```python
from build123d import *

# Parameters (mm, degrees)
F0_R        = 1.5
F1_DEPTH    = 10
F2_DEPTH    = 20
F4_R        = 1.6
F5_DEPTH    = 15
F6_T1_DEPTH = 40
F6_T3_DEPTH = 41.1
F6_T5_DEPTH = 35.7954738485


# Not quite as in the source:
# - a fillet or chamfer that OpenCascade refuses, or shapes differently, is made with other operations: its cross-section is extruded or revolved along the edge and cut away or added


with BuildPart() as f1:
    # F0 (on Top) → F1 (new body)
    with BuildSketch(Plane.XY):
        with BuildLine():
            Line((-15.25, 4.3355262056), (-20.5, 4.5))
            Line((-20.5, 4.5), (-20.5, -4.5))
            Line((-20.5, -4.5), (-10.9144737944, -4.5))
            Line((-10.9144737944, -4.5), (-10.9144737944, 0))
            ThreePointArc((-10.9144737944, 0), (-12.18432002, 3.06567998), (-15.25, 4.3355262056))
        make_face()
        with Locations((-15.25, 0)):
            Circle(F0_R, mode=Mode.SUBTRACT)
        Polygon((20.5, -8.5), (20.5, -4.5), (10.9144737944, -4.5), (-10.9144737944, -4.5), (-20.5, -4.5), (-20.5, -8.5), align=None)
        with BuildLine():
            Line((20.5, -4.5), (20.5, 4.5))
            Line((20.5, 4.5), (15.25, 4.3355262056))
            ThreePointArc((15.25, 4.3355262056), (12.18432002, 3.06567998), (10.9144737944, 0))
            Line((10.9144737944, 0), (10.9144737944, -4.5))
            Line((10.9144737944, -4.5), (20.5, -4.5))
        make_face()
        with Locations((15.25, 0)):
            Circle(F0_R, mode=Mode.SUBTRACT)
    extrude(amount=F1_DEPTH)


with BuildPart() as f2:
    # F0 (on Top) → F2 (new body)
    with BuildSketch(Plane.XY):
        Polygon((20.5, 7.6), (20.5, 4.5), (20.5, -4.5), (20.5, -8.5), (24, -8.5), (24, 0), (24, 7.6), align=None)
    extrude(amount=F2_DEPTH)


with BuildPart() as f1_1:
    add(f1.part)

    # F3: union F2
    add(f2.part)

    # F4 (on face) → F5 (join)
    with BuildSketch(Plane.XZ.offset(8.5)):
        with BuildLine():
            Line((24, 14), (24, 0))
            Line((24, 0), (50, 0))
            Line((50, 0), (50, 14))
            Line((50, 14), (50, 20))
            Line((50, 20), (43.5623936355, 20))
            Line((43.5623936355, 20), (43.5623936355, 14))
            Line((43.5623936355, 14), (43.5, 14))
            ThreePointArc((43.5, 14), (37, 7.5), (30.5, 14))
            Line((30.5, 14), (30.5, 20))
            Line((30.5, 20), (24, 20))
            Line((24, 20), (24, 14))
        make_face()
        with Locations((28, 14)):
            Circle(F4_R, mode=Mode.SUBTRACT)
        with Locations((46, 14)):
            Circle(F4_R, mode=Mode.SUBTRACT)
    extrude(amount=-F5_DEPTH)

    # F6: fillet of radius 5 on 5 edges, made by hand

    # F6_s2 → F6_t1 (cut)
    with BuildSketch(Plane.XZ.offset(-19)):
        with BuildLine():
            ThreePointArc((43.5623936355, 15), (45.0268597296, 18.5355339059), (48.5623936355, 20))
            Line((48.5623936355, 20), (43.5623936355, 20))
            Line((43.5623936355, 20), (43.5623936355, 15))
        make_face()
        with BuildLine():
            ThreePointArc((45, 20), (48.5355339059, 18.5355339059), (50, 15))
            Line((50, 15), (50, 20))
            Line((50, 20), (45, 20))
        make_face()
        with BuildLine():
            ThreePointArc((30.5, 15), (29.0355339059, 18.5355339059), (25.5, 20))
            Line((25.5, 20), (30.5, 20))
            Line((30.5, 20), (30.5, 15))
        make_face()
    extrude(amount=F6_T1_DEPTH, mode=Mode.SUBTRACT)

    # F6_s4 → F6_t3 (cut)
    with BuildSketch(Plane.XZ.offset(-20.1)):
        with BuildLine():
            ThreePointArc((20.5, 15), (21.9644660941, 18.5355339059), (25.5, 20))
            Line((25.5, 20), (20.5, 20))
            Line((20.5, 20), (20.5, 15))
        make_face()
    extrude(amount=F6_T3_DEPTH, mode=Mode.SUBTRACT)

    # F6_s6 → F6_t5 (cut)
    with BuildSketch(Plane.XY.offset(-12.8977369243)):
        with BuildLine():
            ThreePointArc((-20.5, -0.6590947697), (-18.9797396108, 2.9313665155), (-15.3434351037, 4.3384533725))
            Line((-15.3434351037, 4.3384533725), (-20.5, 4.5))
            Line((-20.5, 4.5), (-20.5, -0.6590947697))
        make_face()
    extrude(amount=F6_T5_DEPTH, mode=Mode.SUBTRACT)


solid = f1_1.part
```
Input: part model. Units: mm. Frame: model coordinates. A direction names the side the tool comes from. Round coordinates to 2 decimals unless told otherwise and drop trailing zeros. Loops run counter-clockwise (first coordinate to the right, second up) from the corner with the lowest first, then second, coordinate; pieces in that order, holes last. Notation, with made-up numbers: (-30.5, 1) -> (-20.5, 1) arc R21 ccw to (-20.5, 36) -> close; hole circle Ø6 at (89, 60.5). An arc over 180 degrees is marked (long way). Write each question's results on one line, items separated by ' | '.
1. Section C-C (x = 37). Return loops of the section in (y, z).
Geometry results:
outline: (-8.5, 0) -> (6.5, 0) -> (6.5, 7.5) -> (-8.5, 7.5) -> close
2. Set-up query: faces 1 (the face through (0, -5, 10)), 2 (the face through (-12.15, 3.03, 4.93)), 3 (the face through (44.42, -0.89, 17.8)). Return all of +Z, -Z, +X, -X, +Y, -Y with unobstructed straight access to the full face (end or side cutting, diameter ignored); none if empty.
Geometry results:
face 1: +Z, -X, +Y, -Y | face 2: +Z, -Z, +Y | face 3: +Z, +Y, -Y
3. Section A-A (z = 3.25). Return loops of the section in (x, y), and give its area (3 significant figures).
Geometry results:
outline: (-20.5, -8.5) -> (50, -8.5) -> (50, 6.5) -> (24, 6.5) -> (24, 7.6) -> (20.5, 7.6) -> (20.5, 4.5) -> (15.25, 4.34) arc R4.34 ccw to (10.91, 0) -> (10.91, -4.5) -> (-10.91, -4.5) -> (-10.91, 0) arc R4.34 ccw to (-15.25, 4.34) -> (-15.34, 4.34) arc R5 ccw to (-20.5, -0.66) -> close; hole circle Ø3 at (-15.25, 0); hole circle Ø3 at (15.25, 0) | area: 753 mm2
4. Section D-D (x = -7). Return loops of the section in (y, z), and give its area (3 significant figures).
Geometry results:
outline: (-8.5, 0) -> (-4.5, 0) -> (-4.5, 10) -> (-8.5, 10) -> close | area: 40.0 mm2
5. Section B-B (x = 28). Return loops of the section in (y, z), and give its area (3 significant figures).
Geometry results:
outline: (-8.5, 0) -> (6.5, 0) -> (6.5, 12.4) -> (-8.5, 12.4) -> close; (-8.5, 15.6) -> (6.5, 15.6) -> (6.5, 19.33) -> (-8.5, 19.33) -> close | area: 242 mm2
6. Ray query, line 1 (X direction, y = -4.25, z = 13); line 2 (Y direction, x = -15.25, z = 2); line 3 (X direction, y = 2, z = 14.75). Return the intervals inside material, ascending. Write a range as from..to.
Geometry results:
line 1: 20.5..26.75, 29.25..30.58, 43.42..44.75, 47.25..50 | line 2: -8.5..-1.5, 1.5..4.34 | line 3: 20.5..26.59, 29.41..30.5, 43.56..44.59, 47.41..50
7. First-contact query: P1, Ø1.5, axis at y = 5.5, z = 4.5, coming from the -X side; P2, Ø0.6, axis at y = 7, z = 9.5, coming from the +X side; P3, Ø1.8, axis at x = -15.25, y = 0, coming from the -Z side; P4, Ø5, axis at x = -1, z = 4.5, coming from the +Y side. Flat tips, straight axial feed; report the tip coordinate or a pass-through.
Geometry results:
P1: x = 20.5 | P2: x = 24 | P3: through | P4: y = -4.5
